Design review of the part built by this model. Coordinates are the model's own, in mm. Face numbers are marked on the shaded views. A direction names the side the tool comes from. Coordinates: 2 decimals unless noted, no trailing zeros. Loops run counter-clockwise (first coordinate to the right, second up) from the corner with the lowest first, then second, coordinate; pieces in that order, holes last. Notation, with made-up numbers: M 76.25,-30 L 126.25,-30 A34 cw 126.25,3 Z; hole C -31,59 d10. An arc over 180 degrees is marked long. One line per item, written item: value.
```python
from build123d import *

# Parameters (mm, degrees)
SZKIC1_W                       = 9.9
SZKIC1_H                       = 37
DODANIE_WYCI_GNI_CIE1_DEPTH    = 12.5
DODANIE_WYCI_GNI_CIE2_DEPTH    = 7.5
WYTNIJ_WYCI_GNI_CIE1_START     = -47.15
WYTNIJ_WYCI_GNI_CIE1_OUTLINE_W = 17.51973865
WYTNIJ_WYCI_GNI_CIE1_OUTLINE_H = 49.213267073
WYTNIJ_WYCI_GNI_CIE1_DEPTH     = 47.15
SZKIC4_W                       = 6.3
SZKIC4_H                       = 23.2
WYTNIJ_WYCI_GNI_CIE2_DEPTH     = 57.5
BOSS_EXTRU_1_START             = -2.480261
ESQUISSE2_R                    = 1.8
BOSS_EXTRU_1_DEPTH             = 3
ENL_V_MAT_EXTRU_1_DEPTH        = 72.402310887
ESQUISSE4_W                    = 2.9
ESQUISSE4_H                    = 5.1
ENL_V_MAT_EXTRU_2_DEPTH        = 6.3
BOSS_EXTRU_2_DEPTH             = 37
ESQUISSE6_R                    = 1.1
BOSS_EXTRU_3_DEPTH             = 4.5
ENL_V_START                    = -1.8
ESQUISSE8_R                    = 1.85
ESQUISSE8_R_2                  = 1.1
ENL_V_MAT_EXTRU_5_DEPTH        = 1.8
BOSS_EXTRU_4_REACH             = 76.088
ENL_V_MAT_EXTRU_7_DEPTH        = 75.088410025
ENL_V_MAT_EXTRU_8_DEPTH        = 66.729440163


# Read off the part's stored shape, not the designer's step: Wytnij-wyciągnięcie1
with BuildPart() as part:
    # Szkic1 → Dodanie-wyciągnięcie1 (new body)
    with BuildSketch(Plane(origin=(0, 0, 0), x_dir=(0, 0, -1), z_dir=(1, 0, 0))):
        with Locations((-4.95, 18.5)):
            Rectangle(SZKIC1_W, SZKIC1_H)
    extrude(amount=DODANIE_WYCI_GNI_CIE1_DEPTH)

    # Szkic2 → Dodanie-wyciągnięcie2 (add)
    with BuildSketch(Plane(origin=(12.5, 0, 0), x_dir=(0, 0, -1), z_dir=(1, 0, 0))):
        with BuildLine():
            Line((-45.4, 0), (-7.4, 0))
            Line((-7.4, 0), (-7.4, 37))
            Line((-7.4, 37), (-9.9, 37))
            Line((-9.9, 37), (-55.472391365, 18.25))
            Line((-55.472391365, 18.25), (-57.668539629, -3.378732899))
            ThreePointArc((-57.668539629, -3.378732899), (-51.861031576, -10.142129872), (-45.4, -4))
            Line((-45.4, -4), (-45.4, 0))
        make_face()
    extrude(amount=DODANIE_WYCI_GNI_CIE2_DEPTH)

    # Wytnij-wyciągnięcie1 outline → Wytnij-wyciągnięcie1 (cut)
    with BuildSketch(Plane(origin=(0, 37, 0), x_dir=(1, 0, 0), z_dir=(0, 1, 0)).offset(WYTNIJ_WYCI_GNI_CIE1_START)):
        with Locations((8.759869325, -38.061906093)):
            Rectangle(WYTNIJ_WYCI_GNI_CIE1_OUTLINE_W, WYTNIJ_WYCI_GNI_CIE1_OUTLINE_H)
        Polygon((15, -7.4), (20, -12.4), (20, -7.4), align=None)
    extrude(amount=WYTNIJ_WYCI_GNI_CIE1_DEPTH, mode=Mode.SUBTRACT)

    # Szkic4 → Wytnij-wyciągnięcie2 (cut)
    with BuildSketch(Plane.XY.offset(9.9)):
        with Locations((3.15, 18.5)):
            Rectangle(SZKIC4_W, SZKIC4_H)
    extrude(amount=-WYTNIJ_WYCI_GNI_CIE2_DEPTH, mode=Mode.SUBTRACT)

    # Esquisse2 → Boss.-Extru.1 (add)
    with BuildSketch(Plane(origin=(20, 0, 0), x_dir=(0, 0, -1), z_dir=(1, 0, 0)).offset(BOSS_EXTRU_1_START)):
        with Locations((-51.55, -4)):
            Circle(ESQUISSE2_R)
    extrude(amount=-BOSS_EXTRU_1_DEPTH)

    # Esquisse3 → Enlèv. mat.-Extru.1 (cut, through all)
    with BuildSketch(Plane(origin=(20, 0, 0), x_dir=(0, 0, -1), z_dir=(1, 0, 0))):
        with BuildLine():
            Line((-17.4, 6), (-17.4, 27.014829056))
            ThreePointArc((-17.4, 27.014829056), (-17.843442614, 27.845638225), (-18.780487752, 27.939615015))
            Line((-18.780487752, 27.939615015), (-44.780487752, 17.242348855))
            ThreePointArc((-44.780487752, 17.242348855), (-45.230809169, 16.874120282), (-45.4, 16.317562896))
            Line((-45.4, 16.317562896), (-45.4, 6))
            ThreePointArc((-45.4, 6), (-45.107106781, 5.292893219), (-44.4, 5))
            Line((-44.4, 5), (-18.4, 5))
            ThreePointArc((-18.4, 5), (-17.692893219, 5.292893219), (-17.4, 6))
        make_face()
    extrude(amount=-ENL_V_MAT_EXTRU_1_DEPTH, mode=Mode.SUBTRACT)

    # Esquisse4 → Enlèv. mat.-Extru.2 (cut)
    with BuildSketch(Plane.ZY):
        with Locations((3.95, 32.65)):
            Rectangle(ESQUISSE4_W, ESQUISSE4_H)
        with Locations((3.95, 4.35)):
            Rectangle(ESQUISSE4_W, ESQUISSE4_H)
    extrude(amount=-ENL_V_MAT_EXTRU_2_DEPTH, mode=Mode.SUBTRACT)

    # Esquisse5 → Boss.-Extru.2 (add)
    with BuildSketch(Plane.XZ):
        Polygon((12.5, 4.9), (15, 7.4), (12.5, 7.4), align=None)
    extrude(amount=-BOSS_EXTRU_2_DEPTH)

    # Esquisse6 → Boss.-Extru.3 (add)
    # profile 1 of 3: a face of its own
    with BuildSketch(Plane.ZY):
        Polygon((2.5, 30.1), (2.5, 35.2), (5.4, 35.2), (5.4, 30.1), (9.9, 30.1), (9.9, 37), (0, 37), (0, 30.1), align=None)
    # profile 2 of 3: a face of its own
    with BuildSketch(Plane.ZY):
        with BuildLine():
            ThreePointArc((9.9, 37), (4.95, 41.95), (0, 37))
            Line((0, 37), (9.9, 37))
        make_face()
        with Locations((4.95, 39.475)):
            Circle(ESQUISSE6_R, mode=Mode.SUBTRACT)
    # profile 3 of 3: a face of its own
    with BuildSketch(Plane.ZY):
        with BuildLine():
            ThreePointArc((0, 0), (4.95, -4.95), (9.9, 0))
            Line((9.9, 0), (0, 0))
        make_face()
        with Locations((4.95, -2.475)):
            Circle(ESQUISSE6_R, mode=Mode.SUBTRACT)
    extrude(amount=-BOSS_EXTRU_3_DEPTH)

    # Esquisse8 → Enlèv. mat.-Extru.5 (cut)
    # profile 1 of 2: a face of its own
    with BuildSketch(Plane(origin=(4.5, 0, 0), x_dir=(0, 0, -1), z_dir=(1, 0, 0)).offset(ENL_V_START)):
        with Locations((-4.95, 39.475)):
            Circle(ESQUISSE8_R)
        with Locations(Location((-4.95, 39.475, 0), (0, 0, 180))):
            Circle(ESQUISSE8_R_2, mode=Mode.SUBTRACT)
    # profile 2 of 2: a face of its own
    with BuildSketch(Plane(origin=(4.5, 0, 0), x_dir=(0, 0, -1), z_dir=(1, 0, 0)).offset(ENL_V_START)):
        with Locations((-4.95, -2.475)):
            Circle(ESQUISSE8_R)
        with Locations(Location((-4.95, -2.475, 0), (0, 0, 180))):
            Circle(ESQUISSE8_R_2, mode=Mode.SUBTRACT)
    extrude(amount=ENL_V_MAT_EXTRU_5_DEPTH, mode=Mode.SUBTRACT)

    # Boss.-Extru.4: up to this face of the body (flat: up to its plane)
    boss_extru_4_end = Plane(part.part.faces().sort_by_distance((9.272446383, 37, 5.397564522))[0])
    # Esquisse10 → Boss.-Extru.4 (add, up to the picked face)
    with BuildSketch(Plane.XZ, mode=Mode.PRIVATE) as boss_extru_4_sk1:
        Polygon((20, 0), (12.5, 0), (12.5, 4.9), (20, 12.4), align=None)
    boss_extru_4_tool1 = split(extrude(boss_extru_4_sk1.sketch, amount=-BOSS_EXTRU_4_REACH, mode=Mode.PRIVATE), bisect_by=boss_extru_4_end, keep=Keep.BOTH, mode=Mode.PRIVATE)
    # Esquisse10 → Boss.-Extru.4 (add, up to the picked face)
    with BuildSketch(Plane.XZ, mode=Mode.PRIVATE) as boss_extru_4_sk2:
        Polygon((17.51973865, 13.455272556), (17.51973865, 18.475011205), (12.5, 13.455272556), align=None)
    boss_extru_4_tool2 = split(extrude(boss_extru_4_sk2.sketch, amount=-BOSS_EXTRU_4_REACH, mode=Mode.PRIVATE), bisect_by=boss_extru_4_end, keep=Keep.BOTH, mode=Mode.PRIVATE)
    add(boss_extru_4_tool1.solids().sort_by(Axis((16.791908, 0, 4.595954), (0, 1, 0)))[0])
    add(boss_extru_4_tool2.solids().sort_by(Axis((15.846492, 0, 15.128519), (0, 1, 0)))[0])

    # Esquisse11 → Enlèv. mat.-Extru.7 (cut, through all)
    with BuildSketch(Plane.XZ):
        Polygon((17.51973865, 18.475011205), (18, 18.955272556), (18, 44.91973865), (17.51973865, 45.4), align=None)
        Polygon((12.5, 13.455272556), (12.5, 9.9), (13.509622462, 9.9), (17.51973865, 14.551734777), (17.51973865, 18.475011205), align=None)
        Polygon((17.51973865, 14.551734777), (18, 15.108837944), (18, 18.955272556), (17.51973865, 18.475011205), align=None)
        Polygon((12.5, 4.9), (12.5, 0), (20, 0), (20, 13.6), align=None)
    extrude(amount=-ENL_V_MAT_EXTRU_7_DEPTH, mode=Mode.SUBTRACT)

    # Esquisse12 → Enlèv. mat.-Extru.8 (cut, through all)
    with BuildSketch(Plane(origin=(0, 35.126985948, 14.452412235), x_dir=(1, 0, 0), z_dir=(0, 0.9247859593811136, 0.3804877518811259))):
        Polygon((20, -44.356187196), (20, 0.921740026), (16.810344828, 4.922665822), (13.509622462, 4.922665822), (16.574512596, 1.078238341), (17.51973865, 1.078238341), (17.51973865, -0.107400574), (18, -0.709813663), (18, -32.945273559), (17.51973865, -33.464595187), (17.51973865, -44.356187196), align=None)
        Polygon((16.574512596, 1.078238341), (17.51973865, -0.107400574), (17.51973865, 1.078238341), align=None)
    extrude(amount=ENL_V_MAT_EXTRU_8_DEPTH, mode=Mode.SUBTRACT)


solid = part.part
```
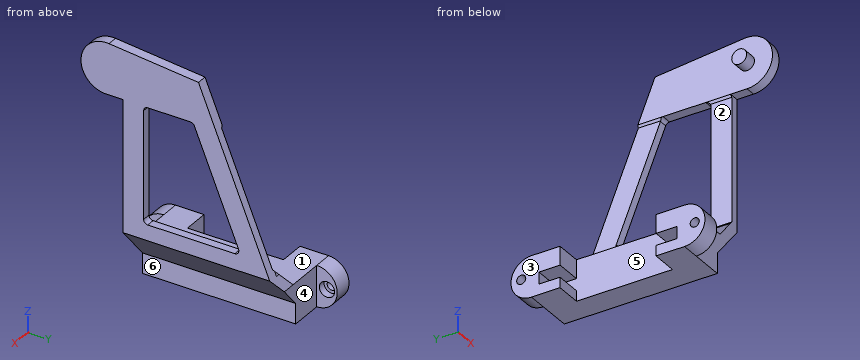
(1) Mouldability with a two-part tool opening along Y and no side actions: class the marked faces 4, 5 and 6 as released by +Y, released by -Y, zero draft, split by the parting line, or undercut.
Reply:
face 4: released by +Y
face 5: undercut
face 6: zero draft
(2) We need section D-D on y = 4. State the section outline as (x, z) points, then the cut area to 3 significant figures.
Reply:
outline: M 0,0 L 12.5,0 L 12.5,4.9 L 20,13.6 L 20,56.92 L 17.52,56.92 L 17.52,45.4 L 18,44.92 L 18,15.11 L 13.51,9.9 L 0,9.9 L 0,5.4 L 6.3,5.4 L 6.3,2.5 L 0,2.5 Z
area: 222 mm2
(3) Tool access review of the marked faces 1, 2 and 3: name each direction out of +Z, -Z, +X, -X, +Y, -Y from which nothing blocks a thin tool from reaching the whole face with its end or side.
Reply:
face 1: +Z, -X, +Y, -Y
face 2: -X, +Y, -Y
face 3: +Z, -Z, -X, +Y, -Y
(4) We need section B-B on y = 31. State the section outline as (x, z) points.
Reply:
outline: M 0,0 L 12.5,0 L 12.5,4.9 L 20,13.6 L 20,24.48 L 18,24.48 L 18,15.11 L 13.51,9.9 L 0,9.9 L 0,5.4 L 6.3,5.4 L 6.3,2.5 L 0,2.5 Z
(5) We need section C-C on x = 10.25. State the section outline as (y, z) points.
Reply:
outline: M 0,0 L 37,0 L 37,9.9 L 0,9.9 Z
(6) We need section A-A on z = 22.5. State the section outline as (x, y) points, then the cut area to 3 significant figures.
Reply:
outline: M 18,0 L 20,0 L 20,5 L 18,5 Z; M 18,26.41 L 20,26.41 L 20,31.82 L 18,31.82 Z
area: 20.8 mm2
(7) Insertion check: pin 1 (1.1 mm diameter, centred on y = -1.5, z = 4.5, fed in from +X); pin 2 (0.8 mm diameter, centred on x = 4, z = 1, fed in from -Y); pin 3 (5.5 mm diameter, centred on y = 11.5, z = 2, fed in from +X). Each pin has a flat end and moves straight along its axis. Give the tip position at first contact, or say it passes through.
Reply:
pin 1: stops at x = 2.7
pin 2: stops at y = -3.45
pin 3: stops at x = 12.5
(8) To check wall thickness, follow line 1 along Y through (x, z) = (1.1, 4.95) (3 decimals); line 2 along Y through (x, z) = (3.55, 4.95) (3 decimals); line 3 along X through (y, z) = (33, 17). State the ranges of each line that lie inside material, in increasing order. Write a range as [from, to].
Reply:
line 1: y = [-4.95, -3.575], [-1.375, 1.8], [35.2, 38.375], [40.575, 41.95]
line 2: y = [-4.95, -4.325], [-0.625, 1.8], [35.2, 37.625], [41.325, 41.95]
line 3: x = [18, 20]
